```python
from build123d import *

# Parameters (mm, degrees)
SKETCH001_R       = 0.35
PAD001_DEPTH      = 10.5
PAD001_DEPTH_BACK = 3.5
SKETCH_R          = 10.5
PAD_DEPTH         = 21
FILLET_R          = 0.5


with BuildPart() as pad001:
    # Sketch001 → Pad001 (new body, two sides)
    with BuildSketch(Plane.XY.offset(0.5)) as pad001_sk:
        Circle(SKETCH001_R)
        with Locations((19, 0)):
            Circle(SKETCH001_R)
    extrude(amount=PAD001_DEPTH)
    extrude(pad001_sk.sketch, amount=-PAD001_DEPTH_BACK)


with BuildPart() as l_radial_d21_0mm_p19_00mm:
    # Sketch → Pad (new body)
    with BuildSketch(Plane.XY.offset(0.1)):
        with Locations((9.5, 0)):
            Circle(SKETCH_R)
    extrude(amount=PAD_DEPTH)

    # Fillet
    fillet_edges = [l_radial_d21_0mm_p19_00mm.edges().sort_by_distance(p)[0] for p in [
        (-1, 0, 0.1),
        (-1, 0, 21.1),
    ]]
    fillet(fillet_edges, radius=FILLET_R)

    add(pad001.part)


solid = l_radial_d21_0mm_p19_00mm.part
```
Model file for the job. Use its own axes, mm. Round coordinates to 2 decimals unless told otherwise and drop trailing zeros. Order: outer loops, then holes, each group sorted by start corner. A loop starts at its lowest first (then second) coordinate and runs counter-clockwise, first axis right, second up. Notation, with made-up numbers: M 74.25,71 L 97.25,71 A31 cw 97.25,102 Z; hole C -11,77 d10. An arc over 180 degrees is marked long. Use CSV: the item, a comma, the result in double quotes.
Item 1: Pin check, flat tips, straight feed: pin 1 (3 mm diameter, centred on y = -3.5, z = 13.5, fed in from +X); pin 2 (5 mm diameter, centred on x = 2, z = 3, fed in from -Y); pin 3 (10 mm diameter, centred on x = 7.5, y = -4, fed in from -Z). Stop position of each tip, or through.
Worked answers:
pin 1,"x = 19.81"
pin 2,"y = -9.23"
pin 3,"z = 0.1"
Item 2: Saw through at A-A (x = 9.5). List the corners of the cut face in (y, z), plus the area to 3 significant figures.
Worked answers:
outline,"M -10.5,0.6 A0.5 ccw -10,0.1 L 10,0.1 A0.5 ccw 10.5,0.6 L 10.5,20.6 A0.5 ccw 10,21.1 L -10,21.1 A0.5 ccw -10.5,20.6 Z"
area,"441 mm²"
Item 3: Probe probe 1 along Y at (x, z) = (9.5, 10.75); probe 2 along Z at (x, y) = (13.5, -5.75); probe 3 along Y at (x, z) = (2, 0.25). List the from-to ranges inside material, lowest first.
Worked answers:
probe 1,"-10.5 to 10.5"
probe 2,"0.1 to 21.1"
probe 3,"-7.14 to 7.14"
Item 4: Saw through at B-B (z = 13.25). List the corners of the cut face in (x, y), plus the area to 3 significant figures.
Worked answers:
outline,"C 9.5,0 d21"
area,"346 mm²"
